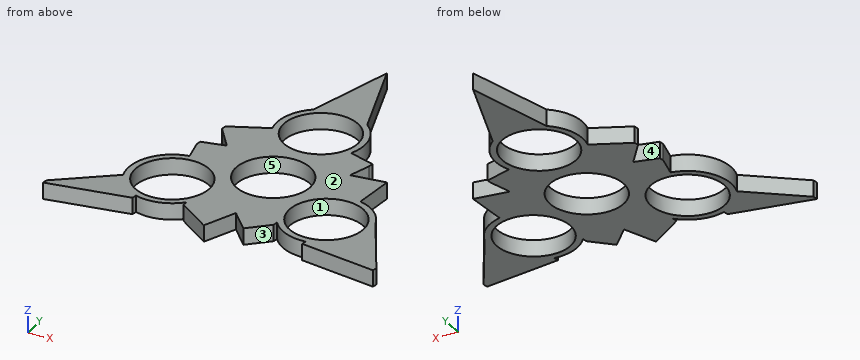
```python
from build123d import *

# Parameters (mm, degrees)
F0_R     = 11.2
F1_DEPTH = 5
F2_DEPTH = 1.5


with BuildPart() as f1:
    # F0 (on Top) → F1 (new body)
    with BuildSketch(Plane.XY):
        with BuildLine():
            Line((19.8292478766, 18.7391326068), (12.019146986, 21.3037386799))
            ThreePointArc((12.019146986, 21.3037386799), (12.8834926091, 29.6341129855), (8.5614465057, 36.807825198))
            ThreePointArc((8.5614465057, 36.807825198), (0.4252472579, 39.9540022295), (-7.8966710373, 37.3383103516))
            ThreePointArc((-7.8966710373, 37.3383103516), (-12.4785048645, 31.0651442851), (-12.7385668251, 23.3012418196))
            Line((-12.7385668251, 23.3012418196), (-24.16729182, 18.2728301734))
            Line((-24.16729182, 18.2728301734), (-17.8012736142, 9.5490273088))
            Line((-17.8012736142, 9.5490273088), (-26.1431888207, 7.8030660957))
            Line((-26.1431888207, 7.8030660957), (-24.4591523854, -0.2429827182))
            ThreePointArc((-24.4591523854, -0.2429827182), (-34.257920026, -6.2095327762), (-35.6854263912, -17.5927569437))
            ThreePointArc((-35.6854263912, -17.5927569437), (-32.5191731961, -22.7044417143), (-27.414141389, -25.8814105115))
            ThreePointArc((-27.414141389, -25.8814105115), (-20.154107372, -26.2299680627), (-13.8101839429, -22.6825433882))
            Line((-13.8101839429, -22.6825433882), (-3.7410892192, -30.0659037435))
            Line((-3.7410892192, -30.0659037435), (0.6309365762, -20.190868824))
            Line((0.6309365762, -20.190868824), (6.3139409441, -26.5421987025))
            Line((6.3139409441, -26.5421987025), (12.4400053994, -21.0607559617))
            ThreePointArc((12.4400053994, -21.0607559617), (17.4984717531, -25.2972406894), (23.9754292514, -26.5561712933))
            ThreePointArc((23.9754292514, -26.5561712933), (34.0938615727, -20.7987226024), (35.7196142534, -9.2710248144))
            ThreePointArc((35.7196142534, -9.2710248144), (32.2340037157, -3.7791277286), (26.5487507681, -0.6186984314))
            Line((26.5487507681, -0.6186984314), (27.9083810392, 11.7930735701))
            Line((27.9083810392, 11.7930735701), (17.170337038, 10.6418415152))
            Line((17.170337038, 10.6418415152), (19.8292478766, 18.7391326068))
        make_face()
        with Locations((-23.1755792411, -13.3804269135)):
            Circle(F0_R, mode=Mode.SUBTRACT)
        with Locations((23.1755792411, -13.3804269135)):
            Circle(F0_R, mode=Mode.SUBTRACT)
        Circle(F0_R, mode=Mode.SUBTRACT)
        with Locations((0, 26.760853827)):
            Circle(F0_R, mode=Mode.SUBTRACT)
        with BuildLine():
            ThreePointArc((-27.414141389, -25.8814105115), (-32.5191731961, -22.7044417143), (-35.6854263912, -17.5927569437))
            Line((-35.6854263912, -17.5927569437), (-52.2249266505, -29.8259742558))
            Line((-52.2249266505, -29.8259742558), (-27.414141389, -25.8814105115))
        make_face()
        with BuildLine():
            Line((47.2735762596, -30.2975326777), (35.7196142534, -9.2710248144))
            ThreePointArc((35.7196142534, -9.2710248144), (34.0938615727, -20.7987226024), (23.9754292514, -26.5561712933))
            Line((23.9754292514, -26.5561712933), (47.2735762596, -30.2975326777))
        make_face()
        with BuildLine():
            ThreePointArc((-7.8966710373, 37.3383103516), (0.4252472579, 39.9540022295), (8.5614465057, 36.807825198))
            Line((8.5614465057, 36.807825198), (0, 63.7780725956))
            Line((0, 63.7780725956), (-7.8966710373, 37.3383103516))
        make_face()
    extrude(amount=F1_DEPTH)

    # F2 (add): faces of the model
    f2_faces = [f1.faces().sort_by_distance(p)[0] for p in [
        (35.6245027555, -28.4268519855, 2.5),
        (41.4965952565, -19.784278746, 2.5),
        (18.4997924573, 14.690487061, 2.5),
        (4.2807232528, 50.2929488968, 2.5),
        (-39.8195340198, -27.8536923837, 2.5),
        (-1.5550763215, -25.1283862838, 2.5),
        (9.3769731717, -23.8014773321, 2.5),
        (-8.775636581, -26.3742235658, 2.5),
        (22.5393590386, 11.2174575427, 2.5),
        (27.2285659036, 5.5871875694, 2.5),
        (3.4724387602, -23.3665337633, 2.5),
        (-25.3011706031, 3.7800416887, 2.5),
        (-20.9842827171, 13.9109287411, 2.5),
        (-3.9483355186, 50.5581914736, 2.5),
        (-18.4529293226, 20.7870359965, 2.5),
        (-21.9722312174, 8.6760467023, 2.5),
        (15.9241974313, 20.0214356434, 2.5),
    ]]
    extrude(f2_faces, amount=F2_DEPTH, dir=(-0.1585548331, -0.9873501734, 0))


solid = f1.part
```
Geometry check sheet. Reference: the model listing, model coordinates, mm. Face numbers are marked on the shaded views. A direction names the side the tool comes from. Give positions to 0.01 mm unless a question says otherwise; leave off trailing zeros. Order: outer loops, then holes, each group sorted by start corner. A loop starts at its lowest first (then second) coordinate and runs counter-clockwise, first axis right, second up.
1. Thickness scan on L1, parallel to Y at x = 9, z = 1.65; L2, parallel to X at y = -3, z = 4.05; L3, parallel to X at y = -5.5, z = 4.4. Record the ranges inside material, lowest first.
2. Section check C-C, the plane y = 46.5. Enter the section's corners in (x, z), and give its area (3 significant figures).
3. Section check B-B, the plane x = -32. Enter the section's corners in (y, z).
4. Gauge pin test, flat ends, axial feed: pin 1 Ø18 at (x, y) = (23.18, -13.38) entering from +Z; pin 2 Ø1.5 at (y, z) = (-0.5, 1) entering from +X. Record the tip position at first contact, or that the pin passes through.
5. Section check D-D, the plane z = 3.85. Give the number of separate pieces and of enclosed holes in the cut face, and give its area (3 significant figures).
6. Release check for a two-part mould opening along Y. For the marked faces 1, 2 and 3 record: pulls with the +Y half, pulls with the -Y half, needs draft (parallel to the pull), parting line crosses it, or undercut.
7. Access from +Z, -Z, +X, -X, +Y, -Y to the whole of each face (thin tool, end or side, straight path). Record for the marked faces 4 and 5.
8. Section check A-A, the plane x = -10. Enter the section's corners in (y, z).
Values follow:
1. L1: y = -25.41 to -6.67, 6.67 to 20.09, 33.43 to 36.42
1. L2: x = -31.33 to -27.38, -18.97 to -10.79, 10.79 to 18.97, 27.38 to 31.33
1. L3: x = -33.77 to -31.13, -15.22 to -9.76, 9.76 to 15.22, 31.13 to 33.77
2. outline: (-5.16, 0) - (5.48, 0) - (5.48, 5) - (-5.16, 5) - close
2. area: 53.2 mm2
3. outline: (-28.05, 0) - (-20.28, 0) - (-20.28, 5) - (-28.05, 5) - close; (-6.48, 0) - (-3.56, 0) - (-3.56, 5) - (-6.48, 5) - close
4. pin 1: passes through
4. pin 2: stops at x = 28.38
5. separate pieces: 1
5. enclosed holes: 4
5. area: 2,090 mm2
6. face 1: undercut
6. face 2: needs draft
6. face 3: pulls with the -Y half
7. face 4: +Z, -Z, -X
7. face 5: +Z, -Z
8. outline: (-27.13, 0) - (-5.04, 0) - (-5.04, 5) - (-27.13, 5) - close; (5.04, 0) - (21.72, 0) - (21.72, 5) - (5.04, 5) - close; (31.8, 0) - (35.38, 0) - (35.38, 5) - (31.8, 5) - close
